Autodesk Inventor part; units mm, degrees
ref_plane "Start plane" through (0, 0, 0) normal (0, 0, 1) x (1, 0, 0)
ref_plane "End plane" through (0, 0, 1800) normal (0, 0, 1) x (1, 0, 0)
ref_plane "YZ Plane" through (0, 0, 0) normal (1, 0, 0) x (0, 1, 0)
ref_plane "Start plane" through (0, 0, 0) normal (0, 0, 1) x (1, 0, 0)
ref_plane "End plane" through (0, 0, 1800) normal (0, 0, 1) x (1, 0, 0)
sketch "Sketch" plane through (0, 0, 0) normal (0, 0, 1) x (1, 0, 0)
  line L0 (-10, -16) -> (-10, 16)
  line L1 (-6, 20) -> (6, 20)
  line L2 (10, 16) -> (10, -16)
  line L3 (6, -20) -> (-6, -20)
  arc A0 (-10, -16) -> (-6, -20) centre (-6, -16) ccw
  arc A1 (10, 16) -> (6, 20) centre (6, 16) ccw
  arc A2 (-6, 20) -> (-10, 16) centre (-6, 16) ccw
  arc A3 (6, -20) -> (10, -16) centre (6, -16) ccw
  arc A4 (-6, 18) -> (-8, 16) centre (-6, 16) ccw
  line L4 (-6, 18) -> (6, 18)
  arc A5 (8, 16) -> (6, 18) centre (6, 16) ccw
  line L5 (8, 16) -> (8, -16)
  arc A6 (6, -18) -> (8, -16) centre (6, -16) ccw
  line L6 (6, -18) -> (-6, -18)
  arc A7 (-8, -16) -> (-6, -18) centre (-6, -16) ccw
  line L7 (-8, -16) -> (-8, 16)
  line L8 (0, 37.1021) -> (0, -37.1021) construction
  line L9 (-23.1021, 0) -> (23.1021, 0) construction
  dimension "d7" = 4
  dimension "d9" = 20
  dimension "d11" = 40
  dimension "d12" = 2
  dimension "d15" = 10
  dimension "d16" = 20
extrude "Body" add sketch "Sketch" along normal up to surface (1800 mm away) from surface at 0
sketch "Sketch3" plane through (0, 0, 0) normal (0, 0, 1) x (1, 0, 0)
  line L0 (0, 0) -> (10, 0)
ref_plane "Work Plane3" through (0, 0, 0) normal (0, -1, 0) x (1, 0, 0)
sketch "Sketch5" plane through (0, 0, 0) normal (1, 0, 0) x (0, 1, 0)
  line L0 (-20, 0) -> (-20, 1800)
  line L1 (-20, 0) -> (-20, 1800)
  line L2 (20, 0) -> (20, 1800)
  line L3 (20, 0) -> (20, 1800)
  line L4 (-20, 0) -> (20, 0)
  line L5 (-20, 1800) -> (20, 1800)
  line L6 (20, 1800) -> (-20, 1771.9917)
  line L7 (20, 0) -> (-20, 57.1259)
  line L8 (-20, 0) -> (-20, 1800)
  point P0 (0, 0)
  dimension "d19" = 55
  dimension "d20" = 35
extrude "Extrusion2" cut sketch "Sketch5" along normal through all both and the other way through all contours L0 L7 L4 | L0 L5 L6
sketch "Sketch4" plane through (0, 0, 0) normal (0, -1, 0) x (1, 0, 0)
  line L0 (-2, 0) -> (12, 0)
  line L1 (-2, 1800) -> (12, 1800)
  dimension "d18" = 1800
equation "\"d7\" = G_IR"
equation "\"d9\" = G_W"
equation "\"d11\" = G_H"
equation "\"d12\" = G_T"
equation "\"d15\" = 0.5 * d9"
equation "\"d16\" = 0.5 * d11"
equation "\"d3\" = G_L"
equation "\"G_W\" = 20"
equation "\"G_H\" = 40"
equation "\"G_T\" = 2"
equation "\"G_IR\" = 4"
equation "\"G_L\" = d18"
equation "\"G_OFFSET_START\" = 0"
equation "\"G_OFFSET_END\" = 0"
properties part number "ISO 4019 - 40x20x2 - 1800" material "Stainless Steel"
The model under review builds one solid part; all positions refer to its coordinate system, in mm. A direction names the side the tool comes from. Round coordinates to 2 decimals unless told otherwise and drop trailing zeros. Order: outer loops, then holes, each group sorted by start corner. A loop starts at its lowest first (then second) coordinate and runs counter-clockwise, first axis right, second up. Notation, with made-up numbers: (3.5, -14.75) - (21.5, -14.75) arc R19 ccw to (21.5, 17.25) - close; hole circle Ø11 at (76, 31). An arc over 180 degrees is marked (long way). Answer in a Markdown table with one row per item.
(1) Take a section at B-B on z = 1547.5. Write out the cut boundary in (x, y), plus the area to 3 significant figures.
Result set:
| item | result |
|---|---|
| outline | (-10, -16) arc R4 ccw to (-6, -20) - (6, -20) arc R4 ccw to (10, -16) - (10, 16) arc R4 ccw to (6, 20) - (-6, 20) arc R4 ccw to (-10, 16) - close; hole (-8, -16) arc R2 ccw to (-6, -18) - (6, -18) arc R2 ccw to (8, -16) - (8, 16) arc R2 ccw to (6, 18) - (-6, 18) arc R2 ccw to (-8, 16) - close |
| area | 214 mm2 |
(2) Clearance check with flat-ended pins moving along their axes: P1, Ø10, axis at x = 7, y = -2, coming from the +Z side; P2, Ø1.5, axis at x = 7, y = 14.5, coming from the +Z side. State where each tip first meets the part, or that it passes through.
Result set:
| item | result |
|---|---|
| P1 | stops at z = 1788.03 |
| P2 | passes through |
(3) Take a section at A-A on x = 2. Write out the cut boundary in (y, z).
Result set:
| item | result |
|---|---|
| outline | (-20, 57.13) - (-18, 54.27) - (-18, 1773.39) - (-20, 1771.99) - close; (18, 2.86) - (20, 0) - (20, 1800) - (18, 1798.6) - close |
(4) Take a section at C-C on y = 0.5. Write out the cut boundary in (x, z), plus the area to 3 significant figures.
Result set:
| item | result |
|---|---|
| outline | (-10, 27.85) - (-8, 27.85) - (-8, 1786.35) - (-10, 1786.35) - close; (8, 27.85) - (10, 27.85) - (10, 1786.35) - (8, 1786.35) - close |
| area | 7,030 mm2 |
(5) Machinability: for faces 1 (the face through (-8.195, 1.575, 1787.099)), 2 (the face through (8, 0, 889)), which of the approach directions +Z, -Z, +X, -X, +Y, -Y give a long, thin tool a straight path to every point of the face, cutting with its end or side? Answer none if there is none.
Result set:
| item | result |
|---|---|
| face 1 | +Z, +X, -X, -Y |
| face 2 | +Z, -Z |
(6) For line 1 (Y direction, x = 6.5, z = 694.5); line 2 (X direction, y = 5.5, z = 818); line 3 (Y direction, x = -5.25, z = 759), list the stretches that pass through material, from the lowest coordinate up. Write a range as from..to.
Result set:
| item | result |
|---|---|
| line 1 | y = -19.97..-17.94, 17.94..19.97 |
| line 2 | x = -10..-8, 8..10 |
| line 3 | y = -20..-18, 18..20 |
